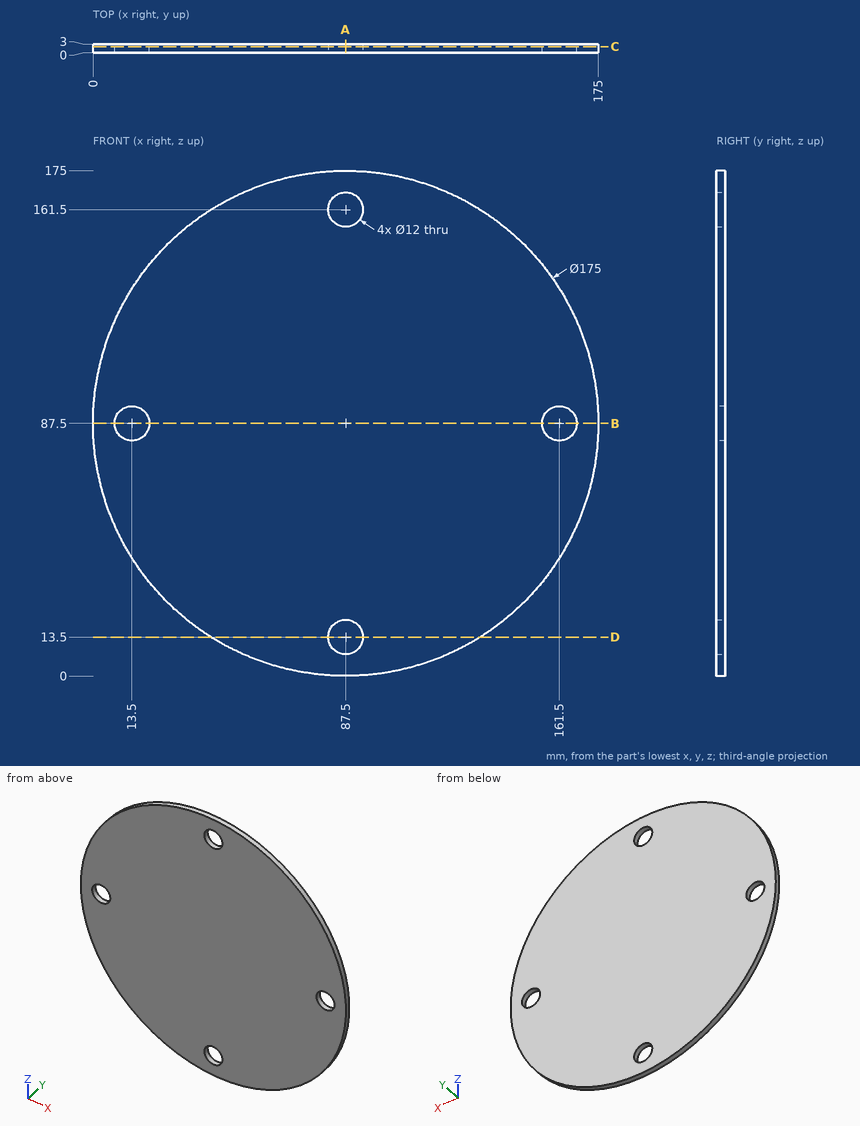
Here's the drawing with two shaded views (mm, measured from the low corner). I have some questions. Round coordinates to 2 decimals unless told otherwise and drop trailing zeros. Loops run counter-clockwise (first coordinate to the right, second up) from the corner with the lowest first, then second, coordinate; pieces in that order, holes last.
Item 1: Suppose I cut it at D-D, the plane z = 13.5. Write out the boundary of the cut face in (x, y).
Item 2: Suppose I cut it at B-B, the plane z = 87.5. Write out the boundary of the cut face in (x, y), then the cut area to 3 significant figures.
Item 3: Please list where these lines run through material, in increasing order: L1, parallel to Z at x = 87.5, y = 1.7; L2, parallel to Z at x = 93, y = 0.7; L3, parallel to Z at x = 161.5, y = 1.75.
Item 4: Will these pins go through, and if not, where does the flat tip stop? pin 1 Ø5 at (x, z) = (130, 58.5) entering from -Y; pin 2 Ø1.5 at (x, y) = (148.5, 2) entering from -Z; pin 3 Ø1 at (y, z) = (2, 120.5) entering from +X.
Item 5: Suppose I cut it at C-C, the plane y = 2.05. Write out the boundary of the cut face in (x, z).
Item 6: Suppose I cut it at A-A, the plane x = 87.5. Write out the boundary of the cut face in (y, z), then the cut area to 3 significant figures.
Reported:
1. outline: (40.81, 0) - (81.5, 0) - (81.5, 3) - (40.81, 3) - close; (93.5, 0) - (134.19, 0) - (134.19, 3) - (93.5, 3) - close
2. outline: (0, 0) - (7.5, 0) - (7.5, 3) - (0, 3) - close; (19.5, 0) - (155.5, 0) - (155.5, 3) - (19.5, 3) - close; (167.5, 0) - (175, 0) - (175, 3) - (167.5, 3) - close
2. area: 453 mm2
3. L1: z = 0 to 7.5, 19.5 to 155.5, 167.5 to 175
3. L2: z = 0.17 to 11.1, 15.9 to 159.1, 163.9 to 174.83
3. L3: z = 40.81 to 81.5, 93.5 to 134.19
4. pin 1: stops at y = 0
4. pin 2: stops at z = 24.05
4. pin 3: stops at x = 168.74
5. outline: circle Ø175 at (87.5, 87.5); hole circle Ø12 at (13.5, 87.5); hole circle Ø12 at (87.5, 13.5); hole circle Ø12 at (87.5, 161.5); hole circle Ø12 at (161.5, 87.5)
6. outline: (0, 0) - (3, 0) - (3, 7.5) - (0, 7.5) - close; (0, 19.5) - (3, 19.5) - (3, 155.5) - (0, 155.5) - close; (0, 167.5) - (3, 167.5) - (3, 175) - (0, 175) - close
6. area: 453 mm2
